Autodesk Inventor part; units mm, degrees
ref_plane "YZ Plane" through (0, 0, 0) normal (1, 0, 0) x (0, 1, 0)
ref_plane "XZ Plane" through (0, 0, 0) normal (0, 1, 0) x (-1, 0, 0)
ref_plane "XY Plane" through (0, 0, 0) normal (0, 0, 1) x (1, 0, 0)
sketch "Esboço1" plane through (0, 0, 0) normal (0, 0, 1) x (1, 0, 0)
  line L0 (-110, 24) -> (110, 24)
  line L1 (110, 24) -> (110, -24)
  line L2 (110, -24) -> (-110, -24)
  line L3 (-110, -24) -> (-110, 24)
  line L4 (-110, 24) -> (110, -24) construction
  line L5 (110, 24) -> (-110, -24) construction
  point P0 (0, 0)
  dimension "d0" = 220
  dimension "d1" = 48
extrude "Extrusão1" add sketch "Esboço1" along normal blind 50
sketch "Esboço2" plane through (-110, -24, 0) normal (-1, 0, 0) x (0, 0, 1)
  line L0 (50, 48) -> (50, 0) construction
  line L1 (0, 48) -> (50, 48) construction
  line L2 (50, 48) -> (50, 0) construction
  line L3 (50, 0) -> (0, 0) construction
  line L4 (0, 0) -> (0, 48) construction
  line L5 (0, 48) -> (50, 0) construction
  line L6 (50, 48) -> (0, 0) construction
  line L7 (0, 48) -> (-20, 48) construction
  line L8 (-20, 48) -> (-20, 0) construction
  line L9 (-20, 0) -> (0, 0) construction
  line L10 (-20, 24) -> (15, 24) construction
  line L11 (50, 48) -> (-20, 48)
  line L12 (-20, 48) -> (-20, 0)
  line L13 (-20, 0) -> (50, 0)
  line L14 (50, 0) -> (50, 48)
  line L15 (50, 48) -> (-20, 0) construction
  line L16 (-20, 48) -> (50, 0) construction
  point P0 (0, 24)
  point P1 (25, 24)
  dimension "d4" = 20
  dimension "d5" = 35
extrude "Extrusão2" add sketch "Esboço2" along normal blind 50
properties part number "ventilador_tangencial_referencia" material "Aço"
Could you check a few things on this model? Use its own coordinates, in mm. A direction names the side the tool comes from. Round coordinates to 2 decimals unless told otherwise and drop trailing zeros. Order: outer loops, then holes, each group sorted by start corner. A loop starts at its lowest first (then second) coordinate and runs counter-clockwise, first axis right, second up.
Q1. Imagine slicing it at A-A, the plane y = 15.5. List the corners of the cut face in (x, z) for me, then the cut area to 3 significant figures.
Geometry says:
outline: (-160, -20) - (-110, -20) - (-110, 0) - (110, 0) - (110, 50) - (-160, 50) - close
area: 14,500 mm2
Q2. Imagine slicing it at B-B, the plane x = -2.5. List the corners of the cut face in (y, z) for me.
Geometry says:
outline: (-24, 0) - (24, 0) - (24, 50) - (-24, 50) - close
Q3. Imagine slicing it at C-C, the plane z = -9.5. List the corners of the cut face in (x, y) for me.
Geometry says:
outline: (-160, -24) - (-110, -24) - (-110, 24) - (-160, 24) - close
Q4. Which directions (+Z, -Z, +X, -X, +Y, -Y) give clear straight access to the entire face, cutting with the end or side of a thin tool? Please do faces 1 (the face through (-2, 0, 0)), 2 (the face through (-160, 0, 15)).
Geometry says:
face 1: -Z, +X, +Y, -Y
face 2: +Z, -Z, -X, +Y, -Y
Q5. Please list where these lines run through material, in increasing order: probe 1 along Z at (x, y) = (91, 19); probe 2 along X at (y, z) = (-9, -16.5).
Geometry says:
probe 1: z = 0 to 50
probe 2: x = -160 to -110
Q6. I'm going to push flat-ended pins straight in: P1, Ø3, axis at y = 14, z = -0.5, coming from the +X side; P2, Ø6, axis at x = 39, y = 2.5, coming from the -Z side. Where does each tip first touch, or does it pass through?
Geometry says:
P1: stops at x = 110
P2: stops at z = 0
